Geometry: final body of the model. Coordinates: model frame, mm. A direction names the side the tool comes from. Give positions to 0.01 mm unless a question says otherwise; leave off trailing zeros. Write each loop counter-clockwise with the first axis right and the second up, starting at its lowest first coordinate (ties: lowest second). Pieces come first, ordered by that corner, then holes.
Autodesk Inventor part; units mm, degrees
ref_plane "YZ Plane" through (0, 0, 0) normal (1, 0, 0) x (0, 1, 0)
ref_plane "XZ Plane" through (0, 0, 0) normal (0, 1, 0) x (-1, 0, 0)
ref_plane "XY Plane" through (0, 0, 0) normal (0, 0, 1) x (1, 0, 0)
sketch "Sketch1" plane through (0, 0, 0) normal (1, 0, 0) x (0, 1, 0)
  line L0 (0, 0) -> (114, 0)
  line L1 (114, 0) -> (114, -50)
  line L2 (0, -50) -> (114, -50)
  line L3 (0, -50) -> (0, 0)
extrude "Extrusion1" add sketch "Sketch1" along normal blind 25
sketch "Sketch2" plane through (25, 0, 0) normal (1, 0, 0) x (0, 0, -1)
  line L0 (50, 114) -> (0, 114)
  line L1 (0, 114) -> (0, 79)
  line L2 (0, 114) -> (0, 0)
  line L3 (50, 0) -> (50, 114)
  line L4 (0, 79) -> (0, 106.71)
  line L5 (50, 79) -> (50, 97.46)
  line L6 (50, 97.46) -> (0, 106.71)
  line L7 (0, 0) -> (50, 0)
  line L8 (0, 106.71) -> (0, 0)
  line L9 (0, 0) -> (50, 0)
  line L10 (50, 0) -> (50, 97.46)
extrude "Extrusion2" add sketch "Sketch2" along normal blind 5 contours L3 L7 L2 L1 L6
mirror "Mirror1" about plane through (30, 51.2546, -24.2418) normal (1, 0, 0) of "Extrusion2", "Extrusion1"
sketch "Sketch3" plane through (0, 0, -50) normal (0, 0, -1) x (-1, 0, 0)
  line L0 (-60, 114) -> (-60, 0)
  line L1 (0, 0) -> (-60, 0)
  line L2 (-60, 0) -> (0, 0)
  line L3 (0, 0) -> (0, 25.8573)
  line L4 (0, 0) -> (0, 114)
  line L5 (-60, 25.8573) -> (0, 25.8573)
  line L6 (-60, 25.8573) -> (-60, 0)
extrude "Extrusion3" add sketch "Sketch3" along normal blind 30
mirror "Mirror2" about plane through (30, 12.9287, -80) normal (0, 0, -1) of "Extrusion2", "Extrusion1", "Mirror1", "Extrusion3"
properties part number "support"
Q1. Section B-B on x = 18. Output: boundary loops of the cut face in (y, z), plus the area to 3 significant figures.
Filled sheet:
outline: (0, -160) - (114, -160) - (114, -110) - (25.86, -110) - (25.86, -50) - (114, -50) - (114, 0) - (0, 0) - close
area: 13,000 mm2
Q2. Pull-direction query (X, two-part tool) for faces 1 (the flat face through (25, 108, -130)), 2 (the flat face through (0, 20, -81)), 3 (the flat face through (35, 107, -130)), 4 (the flat face through (30, 0, -81)); classes: released by +X, released by -X, zero draft, split by the parting line, or undercut.
Filled sheet:
face 1: undercut
face 2: released by -X
face 3: undercut
face 4: zero draft
Q3. Section D-D on y = 102. Output: boundary loops of the cut face in (x, z), plus the area to 3 significant figures.
Filled sheet:
outline: (0, -160) - (60, -160) - (60, -110) - (35, -110) - (35, -134.54) - (25, -134.54) - (25, -110) - (0, -110) - close; (0, -50) - (25, -50) - (25, -25.46) - (35, -25.46) - (35, -50) - (60, -50) - (60, 0) - (0, 0) - close
area: 5,510 mm2
Q4. Ray query, line 1 along Z through (x, y) = (52.5, 95); line 2 along Y through (x, z) = (36.5, -69); line 3 along Y through (x, z) = (28, -152). Return the intervals inside material, ascending.
Filled sheet:
line 1: z = -160 to -110, -50 to 0
line 2: y = 0 to 25.86
line 3: y = 0 to 105.23
Q5. Access query for faces 5 (the flat face through (30, 69, -110)), 6 (the flat face through (48, 114, -135)), 7 (the flat face through (25, 107, -30)). Directions: +Z, -Z, +X, -X, +Y, -Y. A direction counts if a zero-diameter tool reaches every point of the face in a straight line with its end or side. Return the directions, or none.
Filled sheet:
face 5: +X, -X, +Y
face 6: +Z, -Z, +X, -X, +Y
face 7: +Y
Q6. Section C-C on z = -137. Output: boundary loops of the cut face in (x, y) (3 decimals).
Filled sheet:
outline: (0, 0) - (60, 0) - (60, 114) - (35, 114) - (35, 102.455) - (25, 102.455) - (25, 114) - (0, 114) - close
Q7. Pin query (flat end, axial travel): P1, Ø1.5, axis at x = 33.5, z = -117, coming from the +Y side. Return the tip coordinate at first contact, or that it passes through.
Filled sheet:
P1: stops at y = 98.89
Q8. Section A-A on y = 75. Output: boundary loops of the cut face in (x, z).
Filled sheet:
outline: (0, -160) - (60, -160) - (60, -110) - (0, -110) - close; (0, -50) - (60, -50) - (60, 0) - (0, 0) - close
